Here's how the part is built. I have some questions about the finished solid (model axes, mm). A direction names the side the tool comes from. Round coordinates to 2 decimals unless told otherwise and drop trailing zeros. Write each loop counter-clockwise with the first axis right and the second up, starting at its lowest first coordinate (ties: lowest second). Pieces come first, ordered by that corner, then holes. Notation, with made-up numbers: (78.5, 25) -> (112.5, 25) arc R18 cw to (112.5, 60) -> close; hole circle Ø8 at (23, 18.5). An arc over 180 degrees is marked (long way). Answer in a Markdown table with one row per item.
from build123d import *

# Parameters (mm, degrees)
SKETCH_1_R          = 7.5
EXTRUDE_1_DEPTH     = 10
SKETCH_5_W          = 30
SKETCH_5_H          = 52
EXTRUDE_2_DEPTH     = 8
SKETCH_6_W          = 30
SKETCH_6_H          = 8
EXTRUDE_3_DEPTH     = 12
SKETCH_7_R          = 55
EXTRUDE_4_DEPTH     = 8
CUT_EXTRUDE_4_REACH = 40
CUT_EXTRUDE_6_DEPTH = 2
CUT_EXTRUDE_7_REACH = 40
SKETCH_12_R         = 9
SKETCH_13_R         = 10
SKETCH_13_R_2       = 15
CUT_EXTRUDE_8_DEPTH = 10


with BuildPart() as part:
    # 草图1 → 凸台-拉伸1 (new body)
    with BuildSketch(Plane(origin=(0, 0, 0), x_dir=(0, 0, -1), z_dir=(1, 0, 0))):
        Circle(SKETCH_1_R)
    extrude(amount=EXTRUDE_1_DEPTH)

    # 草图5 → 凸台-拉伸2 (add)
    with BuildSketch(Plane(origin=(10, 0, 0), x_dir=(0, 0, -1), z_dir=(1, 0, 0))):
        Rectangle(SKETCH_5_W, SKETCH_5_H)
    extrude(amount=EXTRUDE_2_DEPTH)

    # 草图6 → 凸台-拉伸3 (add)
    with BuildSketch(Plane(origin=(18, 0, 0), x_dir=(0, 0, -1), z_dir=(1, 0, 0))):
        with Locations((0, 22)):
            Rectangle(SKETCH_6_W, SKETCH_6_H)
        with Locations((0, -22)):
            Rectangle(SKETCH_6_W, SKETCH_6_H)
    extrude(amount=EXTRUDE_3_DEPTH)

    # 草图7 → 凸台-拉伸4 (add)
    with BuildSketch(Plane(origin=(30, 0, 0), x_dir=(0, 0, -1), z_dir=(1, 0, 0))):
        Circle(SKETCH_7_R)
    extrude(amount=EXTRUDE_4_DEPTH)

    # 草图8 → 切除-拉伸4 (cut, up to next)
    with BuildSketch(Plane(origin=(38, 0, 0), x_dir=(0, 0, -1), z_dir=(1, 0, 0)), mode=Mode.PRIVATE) as cut_extrude_4_sk1:
        with BuildLine():
            Line((0, 5), (48, 5))
            ThreePointArc((48, 5), (53, 0), (48, -5))
            Line((48, -5), (0, -5))
            ThreePointArc((0, -5), (-5, 0), (0, 5))
        make_face()
    cut_extrude_4_tool1 = extrude(cut_extrude_4_sk1.sketch, amount=-CUT_EXTRUDE_4_REACH, mode=Mode.PRIVATE) & part.part
    add(cut_extrude_4_tool1.solids().sort_by_distance((38, 0, -24))[0], mode=Mode.SUBTRACT)

    # 草图11 → 切除-拉伸6 (cut)
    with BuildSketch(Plane(origin=(38, 0, 0), x_dir=(0, 0, -1), z_dir=(1, 0, 0))):
        with BuildLine():
            Line((0, 7), (54.552726788, 7))
            ThreePointArc((54.552726788, 7), (55, 0), (54.552726788, -7))
            Line((54.552726788, -7), (0, -7))
            ThreePointArc((0, -7), (-7, 0), (0, 7))
        make_face()
    extrude(amount=-CUT_EXTRUDE_6_DEPTH, mode=Mode.SUBTRACT)

    # 草图12 → 切除-拉伸7 (cut, up to next)
    with BuildSketch(Plane.ZY, mode=Mode.PRIVATE) as cut_extrude_7_sk1:
        Circle(SKETCH_12_R)
    cut_extrude_7_tool1 = extrude(cut_extrude_7_sk1.sketch, amount=-CUT_EXTRUDE_7_REACH, mode=Mode.PRIVATE) & part.part
    add(cut_extrude_7_tool1.solids().sort_by_distance((0, 0, 0))[0], mode=Mode.SUBTRACT)

    # 草图13 → 切除-拉伸8 (cut)
    with BuildSketch(Plane.ZY.offset(-30)):
        with Locations((0, 40)):
            Circle(SKETCH_13_R)
        with Locations((35, 0)):
            Circle(SKETCH_13_R_2)
        with Locations((0, -40)):
            Circle(SKETCH_13_R)
    extrude(amount=-CUT_EXTRUDE_8_DEPTH, mode=Mode.SUBTRACT)


solid = part.part
1) I want a section at B-B, the plane z = 1.5. Count the separate pieces of the cut face and the enclosed holes in it, and give its area (3 significant figures).
Response:
| item | result |
|---|---|
| separate pieces | 4 |
| enclosed holes | 0 |
| area | 945 mm^2 |
2) I want a section at D-D, the plane z = 35. List the corners of the cut face in (x, y) for me.
Response:
| item | result |
|---|---|
| outline | (30, -42.43) -> (38, -42.43) -> (38, -15) -> (30, -15) -> close; (30, 15) -> (38, 15) -> (38, 42.43) -> (30, 42.43) -> close |
3) We'd pull the mould along Z, two halves only. Please class faces 4 (the face through (37, 0, 7)), 5 (the face through (33, 0, -53)), 6 (the face through (36, 5.2, -26.4)): +Z half, -Z half, draft (parallel to the pull), parting line (faces both ways), or undercut.
Response:
| item | result |
|---|---|
| face 4 | -Z half |
| face 5 | undercut |
| face 6 | draft |
4) I want a section at C-C, the plane x = 16. List the corners of the cut face in (y, z) for me, and give its area (3 significant figures).
Response:
| item | result |
|---|---|
| outline | (-26, -15) -> (26, -15) -> (26, 15) -> (-26, 15) -> close; hole circle Ø18 at (0, 0) |
| area | 1,310 mm^2 |
5) I need wall thicknesses on line 1 (Y direction, x = 36.25, z = 0); line 2 (Y direction, x = 15.25, z = 0); line 3 (Z direction, x = 31.25, y = -3). Which ranges of each line are inside material? Lowest first, please. Write a range as [from, to].
Response:
| item | result |
|---|---|
| line 1 | y = [-55, -50], [-30, -7], [7, 30], [50, 55] |
| line 2 | y = [-26, -9], [9, 26] |
| line 3 | z = [-54.92, -52], [4, 20.3], [49.7, 54.92] |
6) I want a section at A-A, the plane y = 0. List the corners of the cut face in (x, z) for me.
Response:
| item | result |
|---|---|
| outline | (10, -15) -> (18, -15) -> (18, -9) -> (10, -9) -> close; (10, 9) -> (18, 9) -> (18, 15) -> (10, 15) -> close; (30, -55) -> (36, -55) -> (36, -53) -> (30, -53) -> close; (30, 5) -> (36, 5) -> (36, 7) -> (38, 7) -> (38, 20) -> (30, 20) -> close; (30, 50) -> (38, 50) -> (38, 55) -> (30, 55) -> close |
7) Which directions (+Z, -Z, +X, -X, +Y, -Y) give clear straight access to the entire face, cutting with the end or side of a thin tool? Please do faces 1 (the face through (24, 18, 0)), 2 (the face through (13.944, 8.923, -1.172)), 3 (the face through (33, 5, -24)).
Response:
| item | result |
|---|---|
| face 1 | +Z, -Z |
| face 2 | -X |
| face 3 | +X |
8) For pin 1 (0.6 mm diameter, centred on x = 37.5, z = -36.5, fed in from +Y); pin 2 (4 mm diameter, centred on x = 28.5, z = 19, fed in from +Y); pin 3 (10 mm diameter, centred on x = 35, y = 28, fed in from -Z); pin 4 (16 mm diameter, centred on y = -40, z = 0, fed in from -X), each with a flat end and sliding along its axis, tell me the tip position at first contact or that it passes through.
Response:
| item | result |
|---|---|
| pin 1 | stops at y = 41.41 |
| pin 2 | stops at y = 52.08 |
| pin 3 | stops at z = -49.96 |
| pin 4 | passes through |
